The listing builds one solid part. Answer for the finished solid, in the listing's coordinates (mm). A direction names the side the tool comes from. Coordinates: 2 decimals unless noted, no trailing zeros. Loops run counter-clockwise (first coordinate to the right, second up) from the corner with the lowest first, then second, coordinate; pieces in that order, holes last. Notation, with made-up numbers: (69.5, -6.5) - (117.5, -6.5) arc R14 ccw to (117.5, 0.5) - close; hole circle Ø6 at (75.25, 12.25). An arc over 180 degrees is marked (long way). One line per question, with ' | ' between items.
Autodesk Inventor part; units mm, degrees
ref_plane "YZ Plane" through (0, 0, 0) normal (1, 0, 0) x (0, 1, 0)
ref_plane "XZ Plane" through (0, 0, 0) normal (0, 1, 0) x (-1, 0, 0)
ref_plane "XY Plane" through (0, 0, 0) normal (0, 0, 1) x (1, 0, 0)
sketch "Sketch1" plane through (0, 0, 0) normal (0, 1, 0) x (-1, 0, 0)
  line L0 (0, -57.15) -> (11.43, -57.15)
  line L1 (11.43, -95.25) -> (0, -95.25)
  line L2 (0, -57.15) -> (0, -6.35)
  line L3 (0, -95.25) -> (0, -146.05)
  line L4 (0, -146.05) -> (127, -146.05)
  line L5 (127, -146.05) -> (127, -6.35)
  line L6 (127, -6.35) -> (0, -6.35)
  line L7 (11.43, -17.78) -> (11.43, -45.72)
  line L8 (11.43, -106.68) -> (11.43, -134.62)
  line L9 (11.43, -134.62) -> (115.57, -134.62)
  line L10 (115.57, -134.62) -> (115.57, -17.78)
  line L11 (115.57, -17.78) -> (11.43, -17.78)
  line L12 (11.43, -45.72) -> (11.43, -57.15)
  line L13 (11.43, -106.68) -> (11.43, -95.25)
  point P0 (0, 0)
  dimension "d4" = 50.8
  dimension "d5" = 50.8
  dimension "d6" = 127
  dimension "d7" = 11.43
extrude "Extrusion1" add sketch "Sketch1" along normal blind 6.35
properties part number "Front_chasis"
Item 1: Find the intervals of material crossed by line 1 (Z direction, x = -36, y = 2.75); line 2 (X direction, y = 4.75, z = -41.5); line 3 (X direction, y = 5.25, z = -78.5), in increasing order. Write a range as [from, to].
Taken from the geometry:
line 1: z = [-146.05, -134.62], [-17.78, -6.35] | line 2: x = [-127, -115.57], [-11.43, 0] | line 3: x = [-127, -115.57]
Item 2: Find section C-C, the plane y = 1.5. Write down the section's boundary in (x, z).
Taken from the geometry:
outline: (-127, -146.05) - (0, -146.05) - (0, -95.25) - (-11.43, -95.25) - (-11.43, -134.62) - (-115.57, -134.62) - (-115.57, -17.78) - (-11.43, -17.78) - (-11.43, -57.15) - (0, -57.15) - (0, -6.35) - (-127, -6.35) - close
Item 3: Find section D-D, the plane z = -82.5. Write down the section's boundary in (x, y).
Taken from the geometry:
outline: (-127, 0) - (-115.57, 0) - (-115.57, 6.35) - (-127, 6.35) - close
Item 4: Find section B-B, the plane z = -99. Write down the section's boundary in (x, y).
Taken from the geometry:
outline: (-127, 0) - (-115.57, 0) - (-115.57, 6.35) - (-127, 6.35) - close; (-11.43, 0) - (0, 0) - (0, 6.35) - (-11.43, 6.35) - close
Item 5: The mould has two halves that part along Z. Classify faces 1 (the face through (-63, 3, -146.05)), 2 (the face through (-64, 3, -6.35)), 3 (the face through (-63, 3, -134.62)), 4 (the face through (0, 3, -120)): pulls with the +Z half, pulls with the -Z half, needs draft (parallel to the pull), parting line crosses it, or undercut.
Taken from the geometry:
face 1: pulls with the -Z half | face 2: pulls with the +Z half | face 3: undercut | face 4: needs draft
Item 6: Each of these flat-tipped pins is pushed along its axis until it touches: pin 1 Ø1.9 at (y, z) = (4, -63.5) entering from +X; pin 2 Ø3 at (x, z) = (-87, -131.5) entering from -Y. Where does it stop, or does it pass through?
Taken from the geometry:
pin 1: stops at x = -115.57 | pin 2: passes through
Item 7: Find section A-A, the plane x = -53.5. Write down the section's boundary in (y, z), plus the area to 3 significant figures.
Taken from the geometry:
outline: (0, -146.05) - (6.35, -146.05) - (6.35, -134.62) - (0, -134.62) - close; (0, -17.78) - (6.35, -17.78) - (6.35, -6.35) - (0, -6.35) - close | area: 145 mm2
Item 8: Which of the six approach directions +Z, -Z, +X, -X, +Y, -Y give full straight-line access (tool end or side, diameter ignored) to faces 5 (the face through (-6, 3, -95.25)), 6 (the face through (-64, 3, -17.78)), 7 (the face through (-120, 0, -76))?
Taken from the geometry:
face 5: +X, +Y, -Y | face 6: +Y, -Y | face 7: +Z, -Z, +X, -X, -Y
